Can you work these out from the model? Positions are in its coordinate system, mm. A direction names the side the tool comes from. Coordinates: 2 decimals unless noted, no trailing zeros. Write each loop counter-clockwise with the first axis right and the second up, starting at its lowest first coordinate (ties: lowest second). Pieces come first, ordered by that corner, then holes.
```python
from build123d import *

# Parameters (mm, degrees)
BOSS_EXTRUDE1_DEPTH     = 23.85
SKETCH4_R               = 1.45
CUT_EXTRUDE3_DEPTH      = 10
CUT_EXTRUDE4_DEPTH      = 10
CUT_EXTRUDE4_DEPTH_BACK = 10
SKETCH10_W              = 3.4
SKETCH10_H              = 20


with BuildPart() as part:
    # Sketch1 → Boss-Extrude1 (new body)
    with BuildSketch(Plane.XY):
        with BuildLine():
            Line((-9.1, -10.52892562), (-9.1, 11))
            Line((-9.1, 11), (9.1, 11))
            Line((9.1, 11), (9.1, -11))
            Line((9.1, -11), (9.1, -14))
            Line((9.1, -14), (12.1, -14))
            Line((12.1, -14), (22, -14))
            Line((22, -14), (22, -11))
            Line((22, -11), (15.1, -11))
            ThreePointArc((15.1, -11), (12.978679656, -10.121320344), (12.1, -8))
            Line((12.1, -8), (12.1, 11))
            ThreePointArc((12.1, 11), (11.221320344, 13.121320344), (9.1, 14))
            Line((9.1, 14), (-9.1, 14))
            ThreePointArc((-9.1, 14), (-11.221320344, 13.121320344), (-12.1, 11))
            Line((-12.1, 11), (-12.1, -8))
            ThreePointArc((-12.1, -8), (-12.978679656, -10.121320344), (-15.1, -11))
            Line((-15.1, -11), (-22, -11))
            Line((-22, -11), (-22, -14))
            Line((-22, -14), (-12.1, -14))
            Line((-12.1, -14), (-9.1, -14))
            Line((-9.1, -14), (-9.1, -11))
            Line((-9.1, -11), (-9.507142857, -11))
            Line((-9.507142857, -11), (-9.1, -10.52892562))
        make_face()
    extrude(amount=BOSS_EXTRUDE1_DEPTH)

    # Sketch4 → Cut-Extrude3 (cut)
    with BuildSketch(Plane(origin=(0, -11, 0), x_dir=(1, 0, 0), z_dir=(0, 1, 0))):
        with Locations(Location((-18.55, -21.125, 0), (0, 0, 180))):
            Circle(SKETCH4_R)
        with Locations(Location((-18.55, -2.725, 0), (0, 0, 180))):
            Circle(SKETCH4_R)
        with Locations(Location((18.55, -21.125, 0), (0, 0, 270))):
            Circle(SKETCH4_R)
        with Locations(Location((18.55, -2.725, 0), (0, 0, 180))):
            Circle(SKETCH4_R)
    extrude(amount=-CUT_EXTRUDE3_DEPTH, mode=Mode.SUBTRACT)

    # Sketch10 → Cut-Extrude4 (cut, two sides: drawn at the far end of the back side and taken through both)
    with BuildSketch(Plane.ZY.offset(12.1).offset(-CUT_EXTRUDE4_DEPTH_BACK)):
        with Locations((6.95, -4)):
            Rectangle(SKETCH10_W, SKETCH10_H)
    extrude(amount=CUT_EXTRUDE4_DEPTH + CUT_EXTRUDE4_DEPTH_BACK, mode=Mode.SUBTRACT)


solid = part.part
```
1. If I drill on L1, parallel to Z at x = -18.55, y = -11.95 (3 decimals); L2, parallel to X at y = -5, z = 21.5; L3, parallel to Y at x = 19.5, z = 13.5, over which ranges is the centre line in solid material (lowest first)?
2. I'm going to push flat-ended pins straight in: P1, Ø5, axis at y = 11, z = 21.5, coming from the +X side; P2, Ø8, axis at x = 4.5, y = -6.5, coming from the +Z side; P3, Ø1.6, axis at x = -17.5, z = 3.5, coming from the +Y side; P4, Ø7, axis at y = -1.5, z = 16.5, coming from the -X side. Where does each tip first touch, or does it pass through?
3. If we section it at A-A, the plane y = 2.5: List the corners of the cut face in (x, z) for me, plus the area to 3 significant figures.
4. If we section it at C-C, the plane z = 6: List the corners of the cut face in (x, y) for me, plus the area to 3 significant figures.
5. We'd pull the mould along Z, two halves only. Please class faces 6 (the face through (11.24, 13.1, 11.76)), 7 (the face through (-10, -1, 0)), 8 (the face through (-19.933, -12.479, 3.161)), 9 (the face through (-10, -1, 23.85)): released by +Z, released by -Z, zero draft, split by the parting line, or undercut.
6. Which directions (+Z, -Z, +X, -X, +Y, -Y) give clear straight access to the entire face, cutting with the end or side of a thin tool? Please do faces 1 (the face through (19, -11, 12)), 2 (the face through (15, -14, 12)), 3 (the face through (-11, -6, 8.65)), 4 (the face through (-9.1, 0, 12)), 5 (the face through (-18, -11, 1)).
7. If we section it at B-B, the plane x = -18.55: List the corners of the cut face in (y, z) for me (3 decimals).
8. If we section it at D-D, the plane y = -11.5: List the corners of the cut face in (x, z) for me (3 decimals).
Answers:
1. L1: z = 0 to 1.275, 4.175 to 5.25, 8.65 to 19.675, 22.575 to 23.85
1. L2: x = -12.1 to -9.1, 9.1 to 12.1
1. L3: y = -14 to -11
2. P1: stops at x = 12.1
2. P2: passes through
2. P3: stops at y = -11
2. P4: stops at x = -12.1
3. outline: (-12.1, 0) - (-9.1, 0) - (-9.1, 5.25) - (-12.1, 5.25) - close; (-12.1, 8.65) - (-9.1, 8.65) - (-9.1, 23.85) - (-12.1, 23.85) - close; (9.1, 0) - (12.1, 0) - (12.1, 23.85) - (9.1, 23.85) - close
3. area: 133 mm2
4. outline: (-12.1, 6) - (-9.1, 6) - (-9.1, 11) - (9.1, 11) - (9.1, -14) - (22, -14) - (22, -11) - (15.1, -11) arc R3 cw to (12.1, -8) - (12.1, 11) arc R3 ccw to (9.1, 14) - (-9.1, 14) arc R3 ccw to (-12.1, 11) - close
4. area: 190 mm2
5. face 6: zero draft
5. face 7: released by -Z
5. face 8: undercut
5. face 9: released by +Z
6. face 1: +Z, -Z, +X, +Y
6. face 2: +Z, -Z, +X, -X, -Y
6. face 3: -X, -Y
6. face 4: +Z, -Z, -Y
6. face 5: +Z, -Z, -X, +Y
7. outline: (-14, 0) - (-11, 0) - (-11, 1.275) - (-14, 1.275) - close; (-14, 4.175) - (-11, 4.175) - (-11, 5.25) - (-14, 5.25) - close; (-14, 8.65) - (-11, 8.65) - (-11, 19.675) - (-14, 19.675) - close; (-14, 22.575) - (-11, 22.575) - (-11, 23.85) - (-14, 23.85) - close
8. outline: (-22, 0) - (-9.1, 0) - (-9.1, 5.25) - (-22, 5.25) - close; (-22, 8.65) - (-9.1, 8.65) - (-9.1, 23.85) - (-22, 23.85) - close; (9.1, 0) - (22, 0) - (22, 23.85) - (9.1, 23.85) - close; hole circle Ø2.9 at (-18.55, 2.725); hole circle Ø2.9 at (-18.55, 21.125); hole circle Ø2.9 at (18.55, 2.725); hole circle Ø2.9 at (18.55, 21.125)
